Design review of the part built by this model. Coordinates are the model's own, in mm. Face numbers are marked on the shaded views. A direction names the side the tool comes from. Coordinates: 2 decimals unless noted, no trailing zeros. Order: outer loops, then holes, each group sorted by start corner. A loop starts at its lowest first (then second) coordinate and runs counter-clockwise, first axis right, second up.
from build123d import *

# Parameters (mm, degrees)
BOSS_EXTRUDE2_DEPTH = 10
SKETCH1_5_R         = 2.5
BOSS_EXTRUDE3_DEPTH = 20
CHAMFER1_SIZE       = 10
FILLET1_R           = 5


with BuildPart() as part:
    # Sketch1 → Boss-Extrude2 (new, symmetric)
    with BuildSketch(Plane(origin=(0, 0, 0), x_dir=(0, 0, -1), z_dir=(1, 0, 0))):
        with BuildLine():
            Line((-2.5, -20), (-2.5, -87.425824379))
            ThreePointArc((-2.5, -87.425824379), (-21.281745499, -117.937336386), (12.5, -106))
            Line((12.5, -106), (12.5, -20))
            Line((12.5, -20), (-2.5, -20))
        make_face()
    extrude(amount=BOSS_EXTRUDE2_DEPTH, both=True)

    # Sketch1<5> → Boss-Extrude3 (add, symmetric)
    with BuildSketch(Plane(origin=(0, 0, 0), x_dir=(0, 0, -1), z_dir=(1, 0, 0))):
        Polygon((12.5, -20), (-2.5, -20), (-12.5, -20), (-12.5, 20), (12.5, 20), align=None)
        with Locations((0, 10)):
            Circle(SKETCH1_5_R, mode=Mode.SUBTRACT)
    extrude(amount=BOSS_EXTRUDE3_DEPTH, both=True)

    # Chamfer1
    chamfer1_edges = [part.edges().sort_by_distance(p)[0] for p in [
        (0, -20, 2.5),
    ]]
    chamfer(chamfer1_edges, length=CHAMFER1_SIZE - 0.0001)  # a hair under: the kernel refuses the full size

    # Fillet1
    fillet1_edges = [part.edges().sort_by_distance(p)[0] for p in [
        (10, -117.937336386, 21.281745499),
        (10, -63, -12.5),
        (-10, -58.712862189, 2.5),
        (10, -58.712862189, 2.5),
        (-10, -63, -12.5),
        (-10, -117.937336386, 21.281745499),
        (0, -87.425824379, 2.5),
    ]]
    fillet(fillet1_edges, radius=FILLET1_R)


solid = part.part
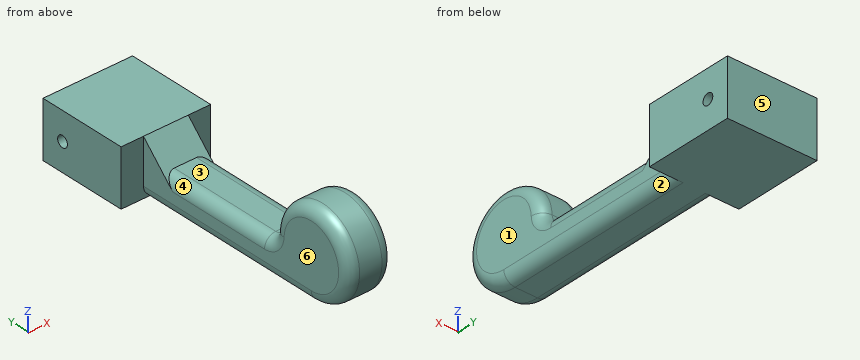
1. For the marked faces 1, 2 and 3, list the 3-axis set-ups (+Z, -Z, +X, -X, +Y, -Y) from which the entire face can be reached by the end or side of a thin tool; tool diameter is ignored.
2. Mouldability with a two-part tool opening along Y and no side actions: class the marked faces 4, 5 and 6 as pulls with the +Y half, pulls with the -Y half, needs draft (parallel to the pull), parting line crosses it, or undercut.
3. Add section C-C (y = -52). Give the boundary of the cut face in (x, z).
4. Add section D-D (x = -16.5). Give the boundary of the cut face in (y, z).
5. Insertion check: pin 1 (8 mm diameter, centred on x = -1, y = -50, fed in from +Z); pin 2 (3 mm diameter, centred on x = -9, y = -35, fed in from +Z); pin 3 (4 mm diameter, centred on y = -75, z = -4.5, fed in from +X); pin 4 (7.5 mm diameter, centred on x = 0.5, z = 3, fed in from -Y). Each pin has a flat end and moves straight along its axis. Give the tip position at first contact, or say it passes through.
6. To check wall thickness, follow line 1 (Y direction, x = -11, z = 0); line 2 (Z direction, x = -5, y = -55.5); line 3 (Y direction, x = -13.5, z = 4). State the ranges of each line that lie inside material, in increasing order.
7. Add section A-A (y = 10). Give the boundary of the cut face in (x, z).
Solution:
1. face 1: +Z, -Z, +X, -Y
1. face 2: -Z, +X, -Y
1. face 3: +Z, +X, -X
2. face 4: undercut
2. face 5: pulls with the +Y half
2. face 6: needs draft
3. outline: (-10, -7.5) arc R5 ccw to (-5, -12.5) - (5, -12.5) arc R5 ccw to (10, -7.5) - (10, -2.5) arc R5 ccw to (5, 2.5) - (-5, 2.5) arc R5 ccw to (-10, -2.5) - close
4. outline: (-20, -12.5) - (20, -12.5) - (20, 12.5) - (-20, 12.5) - close; hole circle Ø5 at (10, 0)
5. pin 1: stops at z = 2.5
5. pin 2: stops at z = 1.83
5. pin 3: stops at x = 10
5. pin 4: stops at y = -125
6. line 1: y = -20 to 7.5, 12.5 to 20
6. line 2: z = -12.5 to 2.5
6. line 3: y = -20 to 20
7. outline: (-20, -12.5) - (20, -12.5) - (20, -2.5) - (-20, -2.5) - close; (-20, 2.5) - (20, 2.5) - (20, 12.5) - (-20, 12.5) - close
